Verification items for the finished model (mm, model axes). Face numbers are marked on the shaded views. A direction names the side the tool comes from. Give positions to 0.01 mm unless a question says otherwise; leave off trailing zeros. Write each loop counter-clockwise with the first axis right and the second up, starting at its lowest first coordinate (ties: lowest second). Pieces come first, ordered by that corner, then holes. Notation, with made-up numbers: (47, -12) -> (67, -12) arc R9 ccw to (67, 0) -> close; hole circle Ø7 at (-12.5, 38.5). An arc over 180 degrees is marked (long way). Write item = value, one per line.
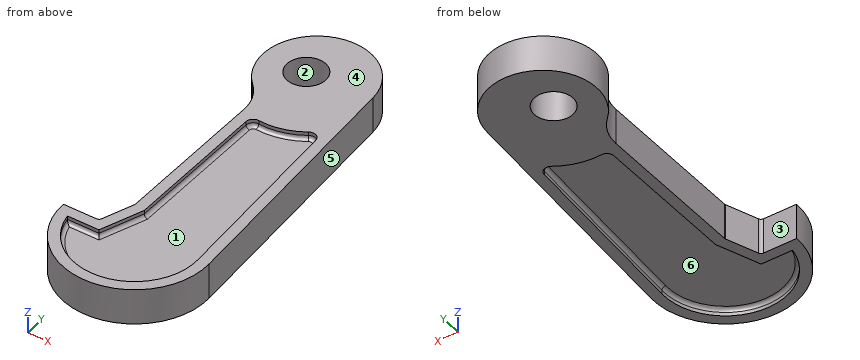
from build123d import *

# Parameters (mm, degrees)
SKETCH2_R           = 5.379907511
BOSS_EXTRUDE1_DEPTH = 5
CUT_EXTRUDE1_DEPTH  = 2
FILLET1_R           = 1
FILLET2_R           = 12


with BuildPart() as part:
    # Sketch2 → Boss-Extrude1 (new body, symmetric)
    with BuildSketch(Plane.XY):
        with BuildLine():
            Line((1.956537451, -8.000102101), (1.956537451, -57.164379656))
            Line((1.956537451, -57.164379656), (-1.463663982, -66.561305864))
            Line((-1.463663982, -66.561305864), (-11.463663982, -66.561305864))
            ThreePointArc((-11.463663982, -66.561305864), (9.219617422, -86.549630619), (28.48964867, -65.195540804))
            Line((28.48964867, -65.195540804), (23.58476107, 6.463017931))
            ThreePointArc((23.58476107, 6.463017931), (0.281599066, 17.907647409), (1.956537451, -8.000102101))
        make_face()
        with Locations((5.619776581, 5.438694136)):
            Circle(SKETCH2_R, mode=Mode.SUBTRACT)
    extrude(amount=BOSS_EXTRUDE1_DEPTH, both=True)

    # Sketch5 → Cut-Extrude1 (cut)
    with BuildSketch(Plane.XY.offset(5)):
        with BuildLine():
            Line((4.956537451, -17.492026764), (4.956537451, -57.693360598))
            Line((4.956537451, -57.693360598), (0.636958632, -69.561305864))
            Line((0.636958632, -69.561305864), (-8.196864513, -69.561305864))
            ThreePointArc((-8.196864513, -69.561305864), (10.619883032, -83.433141325), (25.496651772, -65.400405563))
            Line((25.496651772, -65.400405563), (21.970749815, -13.888307203))
            ThreePointArc((21.970749815, -13.888307203), (20.844130084, -12.223400912), (18.839854353, -12.378525925))
            ThreePointArc((18.839854353, -12.378525925), (13.252017954, -14.955050138), (7.122861364, -15.498954674))
            ThreePointArc((7.122861364, -15.498954674), (5.602404486, -16.020183052), (4.956537451, -17.492026764))
        make_face()
    cut_extrude1 = extrude(amount=-CUT_EXTRUDE1_DEPTH, mode=Mode.SUBTRACT)

    # Mirror1: Cut-Extrude1 across plane
    add(cut_extrude1.mirror(Plane.XY), mode=Mode.SUBTRACT)

    # Fillet1
    fillet1_edges = [part.edges().sort_by_distance(p)[0] for p in [
        (1.956537451, -57.164379656, 0),
        (-1.463663982, -66.561305864, 0),
        (13.252017954, -14.955050138, 3),
        (20.844130084, -12.223400912, 3),
        (23.733700794, -39.644356383, 3),
        (10.619883032, -83.433141325, 3),
        (-3.77995294, -69.561305864, 3),
        (2.796748042, -63.627333231, 3),
        (4.956537451, -37.592693681, 3),
        (5.602404486, -16.020183052, 3),
        (13.252017954, -14.955050138, -3),
        (5.602404486, -16.020183052, -3),
        (4.956537451, -37.592693681, -3),
        (2.796748042, -63.627333231, -3),
        (-3.77995294, -69.561305864, -3),
        (10.619883032, -83.433141325, -3),
        (23.733700794, -39.644356383, -3),
        (20.844130084, -12.223400912, -3),
    ]]
    fillet(fillet1_edges, radius=FILLET1_R)

    # Fillet2
    fillet2_edges = [part.edges().sort_by_distance(p)[0] for p in [
        (1.956537451, -8.000102101, 0),
    ]]
    fillet(fillet2_edges, radius=FILLET2_R)


solid = part.part
Item 1: Sectioned sample at A-A on z = 0.5. Record the cut outline in (x, y).
Response values:
outline = (-11.46, -66.56) arc R20 ccw (long way) to (28.49, -65.2) -> (23.58, 6.46) arc R15 ccw (long way) to (-1.75, -5.4) arc R12 cw to (1.96, -14.07) -> (1.96, -56.99) arc R1 cw to (1.9, -57.33) -> (-1.22, -65.9) arc R1 cw to (-2.16, -66.56) -> close; hole circle Ø10.76 at (5.62, 5.44)
Item 2: Sectioned sample at B-B on x = 26.5. Record the cut outline in (y, z).
Response values:
outline = (-75.35, -5) -> (-36.13, -5) -> (-36.13, 5) -> (-75.35, 5) -> close
Item 3: Material ranges on line 1 (Z direction, x = 6, y = -58.5); line 2 (X direction, y = -70.5, z = 4.25); line 3 (Y direction, x = 8.5, z = 0), recorded low to high.
Response values:
line_1 = -3 to 3
line_2 = -11.07 to -8, 25.07 to 28.14
line_3 = -86.56 to 0.89, 9.98 to 20.44
Item 4: Mould release check, pull along Y, two halves, no side actions. Record for the marked faces 4, 5 and 6: +Y half, -Y half, draft (parallel to the pull), parting line (faces both ways), or undercut.
Response values:
face_4 = draft
face_5 = +Y half
face_6 = undercut
Item 5: Set-up check for the marked faces 1, 2 and 3: record each of +Z, -Z, +X, -X, +Y, -Y from which the full face is reachable in a straight line by a thin tool's end or side.
Response values:
face_1 = +Z
face_2 = +Z, -Z
face_3 = +Z, -Z, -X
Item 6: Sectioned sample at C-C on y = -8. Record the cut outline in (x, z), then the cut area to 3 significant figures.
Response values:
outline = (0.31, -5) -> (24.57, -5) -> (24.57, 5) -> (0.31, 5) -> close
area = 243 mm^2
Item 7: Go/stop test with flat-tipped pins: P1, Ø3, axis at x = 14.5, y = -71, coming from the +Z side; P2, Ø3, axis at y = -20.5, z = -1.5, coming from the +X side; P3, Ø2, axis at x = 2.5, z = 2, coming from the -Y side. Record where each tip stops, or that it passes through.
Response values:
P1 = 3
P2 = 25.53
P3 = -85.92
